from build123d import *

# Parameters (mm, degrees)
SKETCH1_W           = 7.874
SKETCH1_H           = 7.874
SKETCH1_W_2         = 6.35
SKETCH1_H_2         = 6.35
BOSS_EXTRUDE1_DEPTH = 77.999999194
LPATTERN1_COUNT     = 12
LPATTERN1_PITCH     = 7.112
CUT_EXTRUDE1_START  = 3.937
SKETCH3_W           = 86.106
SKETCH3_H           = 77.999999194
CUT_EXTRUDE1_DEPTH  = 0.381


with BuildPart() as part:
    # Sketch1 → Boss-Extrude1 (new body)
    with BuildSketch(Plane(origin=(0, 0, 0), x_dir=(1, 0, 0), z_dir=(0, 1, 0))):
        Rectangle(SKETCH1_W, SKETCH1_H)
        Rectangle(SKETCH1_W_2, SKETCH1_H_2, mode=Mode.SUBTRACT)
    boss_extrude1 = extrude(amount=BOSS_EXTRUDE1_DEPTH)

    # LPattern1: Boss-Extrude1 ×12
    with Locations(*[(i * LPATTERN1_PITCH, 0, 0) for i in range(1, LPATTERN1_COUNT)]):
        add(boss_extrude1)

    # Sketch3 → Cut-Extrude1 (cut)
    with BuildSketch(Plane.XY.offset(CUT_EXTRUDE1_START)):
        with Locations((39.116, 38.999999597)):
            Rectangle(SKETCH3_W, SKETCH3_H)
    extrude(amount=-CUT_EXTRUDE1_DEPTH, mode=Mode.SUBTRACT)


solid = part.part
CAD build for the part. Positions are in the model's coordinates, mm. Round coordinates to 2 decimals unless told otherwise and drop trailing zeros. Loops run counter-clockwise (first coordinate to the right, second up) from the corner with the lowest first, then second, coordinate; pieces in that order, holes last. Notation, with made-up numbers: (56, 68.25) - (67, 68.25) arc R30 ccw to (67, 94.25) - close; hole circle Ø1 at (45.25, 74.5). An arc over 180 degrees is marked (long way). Put each result on its own line as item: value.
1. Slice it at A-A on x = 22.5. List the corners of the cut face in (y, z) (3 decimals).
Geometry check:
outline: (0, -3.937) - (78, -3.937) - (78, -3.175) - (0, -3.175) - close; (0, 3.175) - (78, 3.175) - (78, 3.556) - (0, 3.556) - close
2. Wall check: line 1 (Z direction, x = 24, y = 17.5) (3 decimals). Give the ranges that are in metal, low to high.
Geometry check:
line 1: -3.937 to -3.175, 3.175 to 3.556
3. Two-plate mould, pull along Z, no slides. Class faces 1 (the flat face through (64, 38, 3.175)), 2 (the flat face through (-3.937, 38, 0)), 3 (the flat face through (39, 38, -3.937)): released by +Z, released by -Z, zero draft, split by the parting line, or undercut.
Geometry check:
face 1: undercut
face 2: zero draft
face 3: released by -Z
4. Slice it at B-B on z = -0.5. Give the number of separate pieces and of enclosed holes in the cut face, and give its area (3 significant figures).
Geometry check:
separate pieces: 13
enclosed holes: 0
area: 773 mm²
